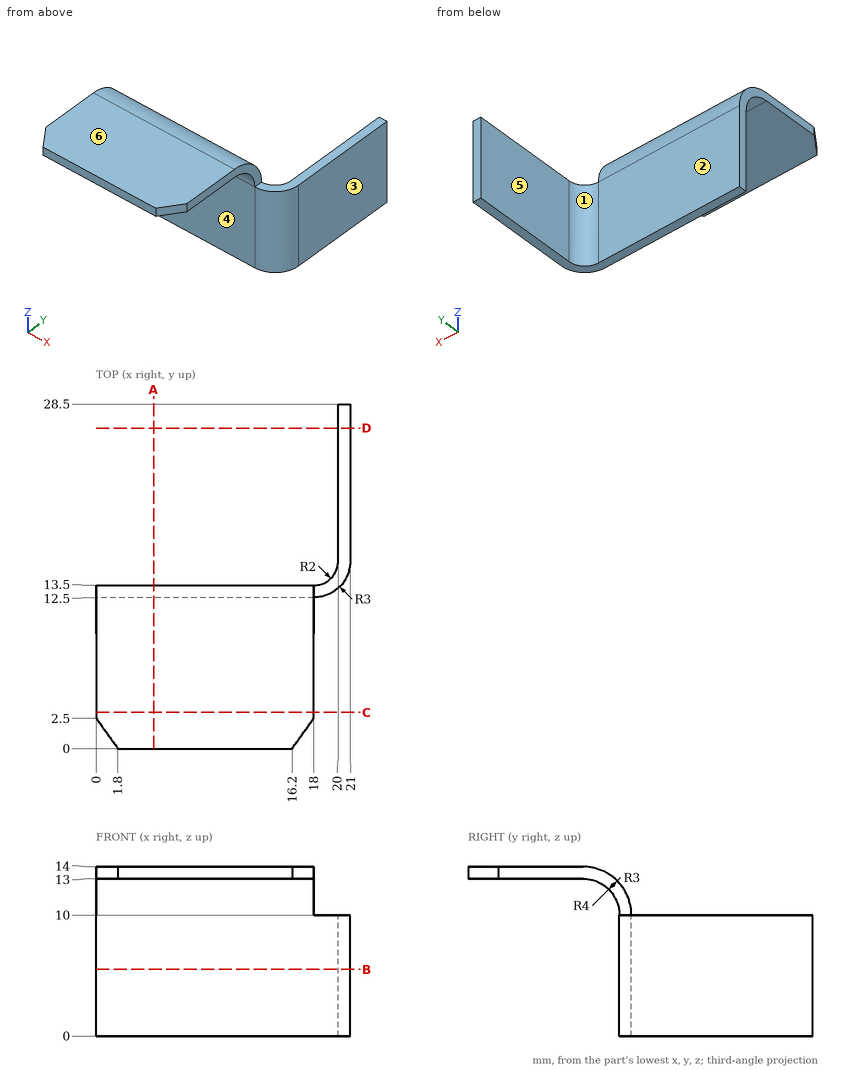
Here's the drawing with two shaded views (mm, measured from the low corner). I have some questions. A direction names the side the tool comes from. Coordinates: 2 decimals unless noted, no trailing zeros. Write each loop counter-clockwise with the first axis right and the second up, starting at its lowest first coordinate (ties: lowest second). Pieces come first, ordered by that corner, then holes. Notation, with made-up numbers: (-31, 17.5) -> (11, 17.5) arc R19 cw to (11, 40.5) -> close; hole circle Ø10 at (-33, 53). An arc over 180 degrees is marked (long way). Write item = value, one per line. Start each with the question number.
(1) We'd pull the mould along X, two halves only. Please class the marked faces 1, 2 and 3: released by +X, released by -X, zero draft, split by the parting line, or undercut.
(2) I want a section at B-B (z = 5.5). Please give me the cut outline in (x, y), plus the area to 3 significant figures.
(3) I need wall thicknesses on line 1 (Y direction, x = 6.5, z = 8.25); line 2 (Z direction, x = 5.25, y = 7.75); line 3 (X direction, y = 23.5, z = 5.25). Which ranges of each line are inside material? Lowest first, please. Write a range as [from, to].
(4) Which directions (+Z, -Z, +X, -X, +Y, -Y) give clear straight access to the entire face, cutting with the end or side of a thin tool? Please do the marked faces 4, 5 and 6.
(5) I want a section at C-C (y = 3). Please give me the cut outline in (x, z).
(6) Will these pins go through, and if not, where does the flat tip stop? pin 1 (12 mm diameter, centred on x = 4.5, y = 10, fed in from -Z); pin 2 (2.5 mm diameter, centred on x = 19, y = 24.5, fed in from +Z); pin 3 (3 mm diameter, centred on x = 8, z = 3, fed in from +Y); pin 4 (2 mm diameter, centred on x = 17.5, y = 3.5, fed in from -Z).
(7) I want a section at D-D (y = 26.5). Please give me the cut outline in (x, z), plus the area to 3 significant figures.
(8) I want a section at A-A (x = 4.75). Please give me the cut outline in (y, z), plus the area to 3 significant figures.
Result set:
q1.face_1 = released by -X
q1.face_2 = zero draft
q1.face_3 = released by +X
q2.outline = (0, 12.5) -> (18, 12.5) arc R3 ccw to (21, 15.5) -> (21, 28.5) -> (20, 28.5) -> (20, 15.5) arc R2 cw to (18, 13.5) -> (0, 13.5) -> close
q2.area = 34.9 mm2
q3.line_1 = [12.5, 13.5]
q3.line_2 = [13, 14]
q3.line_3 = [20, 21]
q4.face_4 = -Z, +X, -X, -Y
q4.face_5 = +Z, -Z, -X, +Y
q4.face_6 = +Z, +X, -X, +Y, -Y
q5.outline = (0, 13) -> (18, 13) -> (18, 14) -> (0, 14) -> close
q6.pin_1 = 0
q6.pin_2 = 10
q6.pin_3 = 13.5
q6.pin_4 = 13
q7.outline = (20, 0) -> (21, 0) -> (21, 10) -> (20, 10) -> close
q7.area = 10.0 mm2
q8.outline = (0, 13) -> (9.5, 13) arc R3 cw to (12.5, 10) -> (12.5, 0) -> (13.5, 0) -> (13.5, 10) arc R4 ccw to (9.5, 14) -> (0, 14) -> close
q8.area = 25.0 mm2
